```python
from build123d import *

# Parameters (mm, degrees)
SKETCH1_W           = 28.2
SKETCH1_H           = 29.2
BOSS_EXTRUDE1_DEPTH = 3
BOSS_EXTRUDE2_START = -3
SKETCH1_3_W         = 28.2
SKETCH1_3_H         = 29.2
BOSS_EXTRUDE2_DEPTH = 30
SKETCH3_3_W         = 20.4
SKETCH3_3_H         = 20.4
CUT_EXTRUDE1_DEPTH  = 30
CUT_EXTRUDE2_REACH  = 72.378
SKETCH4_R           = 2


with BuildPart() as part:
    # Sketch1 → Boss-Extrude1 (new body)
    with BuildSketch(Plane.XY):
        with Locations((-1, 0)):
            Rectangle(SKETCH1_W, SKETCH1_H)
    boss_extrude1 = extrude(amount=-BOSS_EXTRUDE1_DEPTH)

    # Sketch1<3> → Boss-Extrude2 (add)
    with BuildSketch(Plane.XY.offset(BOSS_EXTRUDE2_START)):
        with Locations((-1, 0)):
            Rectangle(SKETCH1_3_W, SKETCH1_3_H)
        with BuildLine():
            Line((-10.1, 2.9), (-10.1, 9))
            ThreePointArc((-10.1, 9), (-9.777817459, 9.777817459), (-9, 10.1))
            Line((-9, 10.1), (-2.9, 10.1))
            Line((-2.9, 10.1), (-2.9, 7.9))
            Line((-2.9, 7.9), (-4.9, 7.9))
            Line((-4.9, 7.9), (-4.9, 5.749))
            Line((-4.9, 5.749), (-2.7515, 3.6005))
            Line((-2.7515, 3.6005), (2.7515, 3.6005))
            Line((2.7515, 3.6005), (4.9, 5.749))
            Line((4.9, 5.749), (4.9, 7.9))
            Line((4.9, 7.9), (2.9, 7.9))
            Line((2.9, 7.9), (2.9, 10.1))
            Line((2.9, 10.1), (9, 10.1))
            ThreePointArc((9, 10.1), (9.777817459, 9.777817459), (10.1, 9))
            Line((10.1, 9), (10.1, 2.9))
            Line((10.1, 2.9), (7.9, 2.9))
            Line((7.9, 2.9), (7.9, 4.9))
            Line((7.9, 4.9), (5.749, 4.9))
            Line((5.749, 4.9), (3.6005, 2.7515))
            Line((3.6005, 2.7515), (3.6005, -2.7515))
            Line((3.6005, -2.7515), (5.749, -4.9))
            Line((5.749, -4.9), (7.9, -4.9))
            Line((7.9, -4.9), (7.9, -2.9))
            Line((7.9, -2.9), (10.1, -2.9))
            Line((10.1, -2.9), (10.1, -9))
            ThreePointArc((10.1, -9), (9.777817459, -9.777817459), (9, -10.1))
            Line((9, -10.1), (2.9, -10.1))
            Line((2.9, -10.1), (2.9, -7.9))
            Line((2.9, -7.9), (4.9, -7.9))
            Line((4.9, -7.9), (4.9, -5.749))
            Line((4.9, -5.749), (2.7515, -3.6005))
            Line((2.7515, -3.6005), (-2.7515, -3.6005))
            Line((-2.7515, -3.6005), (-4.9, -5.749))
            Line((-4.9, -5.749), (-4.9, -7.9))
            Line((-4.9, -7.9), (-2.9, -7.9))
            Line((-2.9, -7.9), (-2.9, -10.1))
            Line((-2.9, -10.1), (-9, -10.1))
            ThreePointArc((-9, -10.1), (-9.777817459, -9.777817459), (-10.1, -9))
            Line((-10.1, -9), (-10.1, -2.9))
            Line((-10.1, -2.9), (-7.9, -2.9))
            Line((-7.9, -2.9), (-7.9, -4.9))
            Line((-7.9, -4.9), (-5.749, -4.9))
            Line((-5.749, -4.9), (-3.6005, -2.7515))
            Line((-3.6005, -2.7515), (-3.6005, 2.7515))
            Line((-3.6005, 2.7515), (-5.749, 4.9))
            Line((-5.749, 4.9), (-7.9, 4.9))
            Line((-7.9, 4.9), (-7.9, 2.9))
            Line((-7.9, 2.9), (-10.1, 2.9))
        make_face(mode=Mode.SUBTRACT)
    boss_extrude2 = extrude(amount=-BOSS_EXTRUDE2_DEPTH)

    # Mirror1: Boss-Extrude1, Boss-Extrude2 across plane
    add(boss_extrude1.mirror(Plane(origin=(-15.1, 0, -3), x_dir=(0, 0, 1), z_dir=(-1, 0, 0))))
    add(boss_extrude2.mirror(Plane(origin=(-15.1, 0, -3), x_dir=(0, 0, 1), z_dir=(-1, 0, 0))))

    # Sketch3 → section 1 of loft1
    with BuildSketch(Plane(origin=(0, -44.6, 0), x_dir=(-1, 0, 0), z_dir=(0, -1, 0)), mode=Mode.PRIVATE) as loft1_s1:
        with BuildLine():
            Line((2.1, 7), (28.1, 7))
            Line((28.1, 7), (28.1, 33))
            Line((28.1, 33), (2.1, 33))
            Line((2.1, 33), (2.1, 7))
        make_face()
    # loft from a face of the part (loft1)
    loft([part.faces().sort_by_distance((-15.1, -14.6, -16.5))[0], loft1_s1.sketch])

    # Sketch3<3> → Cut-Extrude1 (cut)
    with BuildSketch(Plane(origin=(0, -44.6, 0), x_dir=(-1, 0, 0), z_dir=(0, -1, 0))):
        with Locations((15.1, 20)):
            Rectangle(SKETCH3_3_W, SKETCH3_3_H)
    extrude(amount=-CUT_EXTRUDE1_DEPTH, mode=Mode.SUBTRACT)

    # Sketch4 → Cut-Extrude2 (cut, up to next)
    with BuildSketch(Plane(origin=(0, 0, -33), x_dir=(-1, 0, 0), z_dir=(0, 0, -1)), mode=Mode.PRIVATE) as cut_extrude2_sk1:
        with Locations((15.1, -37.1)):
            Circle(SKETCH4_R)
    cut_extrude2_tool1 = extrude(cut_extrude2_sk1.sketch, amount=-CUT_EXTRUDE2_REACH, mode=Mode.PRIVATE) & part.part
    # Sketch4 → Cut-Extrude2 (cut, up to next)
    with BuildSketch(Plane(origin=(0, 0, -33), x_dir=(-1, 0, 0), z_dir=(0, 0, -1)), mode=Mode.PRIVATE) as cut_extrude2_sk2:
        with Locations((15.1, -22.1)):
            Circle(SKETCH4_R)
    cut_extrude2_tool2 = extrude(cut_extrude2_sk2.sketch, amount=-CUT_EXTRUDE2_REACH, mode=Mode.PRIVATE) & part.part
    add(cut_extrude2_tool1.solids().sort_by_distance((-15.1, -37.1, -33))[0], mode=Mode.SUBTRACT)
    add(cut_extrude2_tool2.solids().sort_by_distance((-15.1, -22.1, -33))[0], mode=Mode.SUBTRACT)


solid = part.part
```
Input: part model. Units: mm. Frame: model coordinates. A direction names the side the tool comes from. Coordinates: 2 decimals unless noted, no trailing zeros. Use a Markdown table: item, result. Add a question column.
1) Set-up query: faces 1 (the flat face through (-15, -30, -30.2)), 2 (the flat face through (-25.51, -3.84, -17.79)). Return all of +Z, -Z, +X, -X, +Y, -Y with unobstructed straight access to the full face (end or side cutting, diameter ignored); none if empty.
2) Line query: L1, parallel to Y at x = -15, z = -32; L2, parallel to X at y = 1, z = -21.5; L3, parallel to Y at x = -8, z = -19. Output: solid intervals per line, ascending. Write a range as from..to.
3) Pin query (flat end, axial travel): P1, Ø1.5, axis at y = -15.5, z = -27.5, coming from the -X side; P2, Ø5, axis at x = 7.5, z = -13.5, coming from the -Y side; P3, Ø2.5, axis at x = -6.5, z = -11.5, coming from the -Y side; P4, Ø4, axis at x = -30.5, y = -3, coming from the -Z side. Return the tip coordinate at first contact, or that it passes through.
4) Draft query along Z for faces 3 (the flat face through (-15, 0, 0)), 4 (the flat face through (-4, -7.9, -18)), 5 (the flat face through (-4.9, -30, -20)). Return one class per face: +Z half, -Z half, draft (parallel to the pull), parting line (faces both ways), or undercut.
5) Section A-A, the plane z = -8. Give the number of separate pieces and of enclosed holes in the cut face, plus the area to 3 significant figures.
Answer below:
| question | item | result |
|---|---|---|
| 1 | face 1 | -Y |
| 1 | face 2 | -Z |
| 2 | L1 | -44.6..-39.1, -35.1..-24.1, -20.1..14.6 |
| 2 | L2 | -43.3..-33.8, -26.6..-3.6, 3.6..13.1 |
| 2 | L3 | -14.6..-10.1, -2.9..2.9, 10.1..14.6 |
| 3 | P1 | x = -43.22 |
| 3 | P2 | y = -30.59 |
| 3 | P3 | y = -14.6 |
| 3 | P4 | z = -33 |
| 4 | face 3 | +Z half |
| 4 | face 4 | draft |
| 4 | face 5 | undercut |
| 5 | separate pieces | 1 |
| 5 | enclosed holes | 2 |
| 5 | area | 2,470 mm2 |
